from build123d import *

# Parameters (mm, degrees)
BOX015_W          = 8.4
BOX015_H          = 1.2
BOX015_DEPTH      = 3
CYLINDER069_R     = 1.5
CYLINDER069_DEPTH = 8
CYLINDER064_R     = 4
CYLINDER064_DEPTH = 11


with BuildPart() as pick_slot:
    # Box015 → Box015 (new body)
    with BuildSketch(Plane(origin=(-4.2, -0.6, 8), x_dir=(1, 0, 0), z_dir=(0, 0, 1))):
        with Locations((4.2, 0.6)):
            Rectangle(BOX015_W, BOX015_H)
    extrude(amount=BOX015_DEPTH)


with BuildPart() as axis_hole:
    # Cylinder069 → Cylinder069 (new body)
    with BuildSketch(Plane.XY):
        Circle(CYLINDER069_R)
    extrude(amount=CYLINDER069_DEPTH)


with BuildPart() as pot_axis_ext:
    # Cylinder064 → Cylinder064 (new body)
    with BuildSketch(Plane.XY):
        Circle(CYLINDER064_R)
    extrude(amount=CYLINDER064_DEPTH)

    # Cut051: cut axis-hole
    add(axis_hole.part, mode=Mode.SUBTRACT)

    # Cut052: cut pick-slot
    add(pick_slot.part, mode=Mode.SUBTRACT)


with BuildPart() as pot_axis_ext_1:
    # Cut052 placement: moved
    add(pot_axis_ext.part.moved(Location((0, 0, 40.2))))


solid = pot_axis_ext_1.part
Work out the finished part from the listing and answer in its coordinate system (mm). A direction names the side the tool comes from. Round coordinates to 2 decimals unless told otherwise and drop trailing zeros. Loops run counter-clockwise (first coordinate to the right, second up) from the corner with the lowest first, then second, coordinate; pieces in that order, holes last. Notation, with made-up numbers: (44.25, 24.25) - (66.25, 24.25) arc R23 ccw to (66.25, 49.25) - close; hole circle Ø3 at (65.25, -37). An arc over 180 degrees is marked (long way). One line per item, written item: value.
Q1. Find section C-C on z = 45.5. Give the vertices of the cut face in (x, y), and give its area (3 significant figures).
Check values:
outline: circle Ø8 at (0, 0); hole circle Ø3 at (0, 0)
area: 43.2 mm2
Q2. Each of these flat-tipped pins is pushed along its axis until it touches: pin 1 Ø2.5 at (x, y) = (0, 0) entering from -Z; pin 2 Ø1.5 at (y, z) = (-2, 44.5) entering from +X; pin 3 Ø1 at (x, y) = (3, 0) entering from +Z. Where does it stop, or does it pass through?
Check values:
pin 1: z = 48.2
pin 2: x = 3.8
pin 3: z = 48.2
Q3. For faces 4 (the cylindrical face through (-1.5, 0.07, 44.14)), 5 (the flat face through (0, 2, 51.2)), 6 (the flat face through (3, 0, 48.2)), determine the directions among +Z, -Z, +X, -X, +Y, -Y from which every point of the face is accessible in a straight line to the end or side of a thin tool.
Check values:
face 4: -Z
face 5: +Z, +X, -X, +Y, -Y
face 6: +Z, +X, -X
Q4. The mould has two halves that part along X. Classify faces 1 (the flat face through (0, -1, 48.2)), 2 (the flat face through (-3, 0, 48.2)), 3 (the cylindrical face through (3.695, -1.532, 45.623)): +X half, -X half, draft (parallel to the pull), parting line (faces both ways), or undercut.
Check values:
face 1: undercut
face 2: draft
face 3: parting line
Q5. Straight lines are drawn through the part: probe 1 along Y at (x, z) = (0, 45.75); probe 2 along Y at (x, z) = (3.25, 48.25); probe 3 along Z at (x, y) = (-2.25, 0.25). For each, find the intervals that lie inside material, in ascending order.
Check values:
probe 1: -4 to -1.5, 1.5 to 4
probe 2: -2.33 to -0.6, 0.6 to 2.33
probe 3: 40.2 to 48.2
Q6. Find section B-B on x = 0. Give the vertices of the cut face in (y, z), and give its area (3 significant figures).
Check values:
outline: (-4, 40.2) - (-1.5, 40.2) - (-1.5, 48.2) - (-0.6, 48.2) - (-0.6, 51.2) - (-4, 51.2) - close; (0.6, 48.2) - (1.5, 48.2) - (1.5, 40.2) - (4, 40.2) - (4, 51.2) - (0.6, 51.2) - close
area: 60.4 mm2
Q7. Find section D-D on z = 49.25. Give the vertices of the cut face in (x, y).
Check values:
outline: (-3.95, -0.6) arc R4 ccw to (3.95, -0.6) - close; (-3.95, 0.6) - (3.95, 0.6) arc R4 ccw to start
Q8. Find section A-A on y = 0. Give the vertices of the cut face in (x, z).
Check values:
outline: (-4, 40.2) - (-1.5, 40.2) - (-1.5, 48.2) - (-4, 48.2) - close; (1.5, 40.2) - (4, 40.2) - (4, 48.2) - (1.5, 48.2) - close
